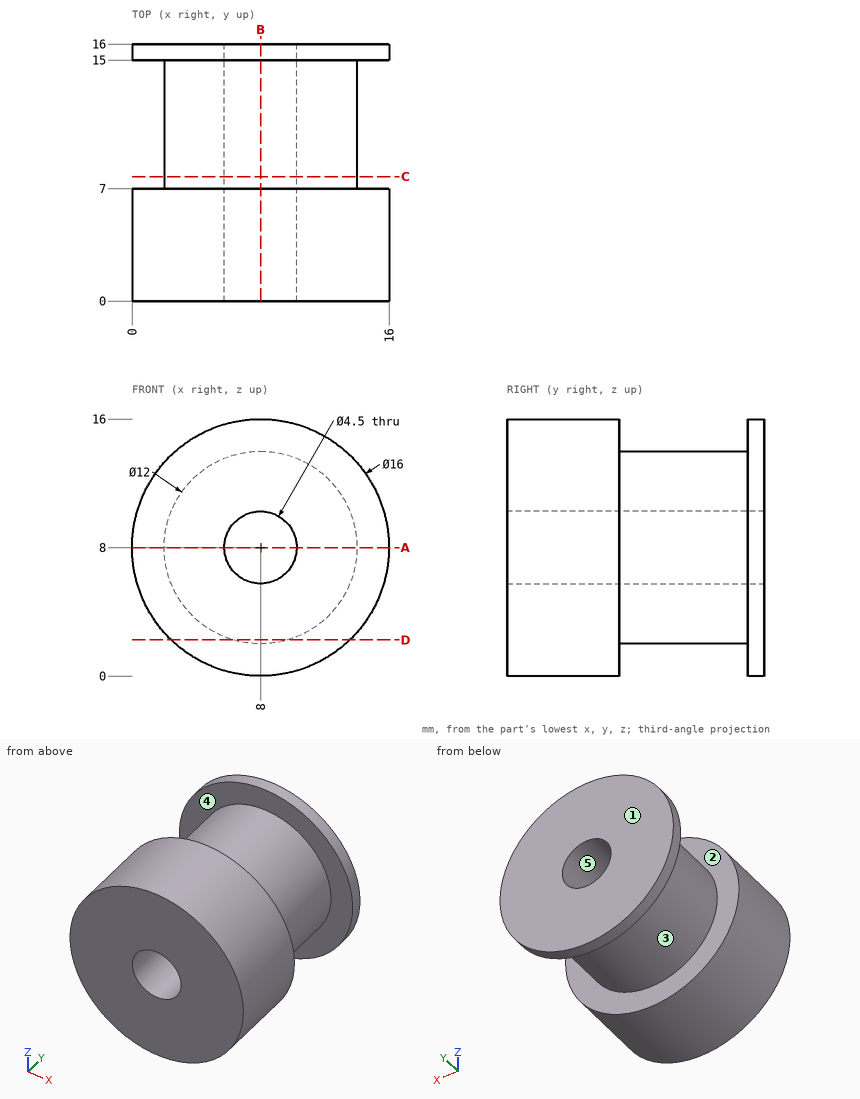
Verification items for this drawing (mm, ordinates from the low corner). A direction names the side the tool comes from. Give positions to 0.01 mm unless a question says otherwise; leave off trailing zeros. Write each loop counter-clockwise with the first axis right and the second up, starting at its lowest first coordinate (ties: lowest second). Pieces come first, ordered by that corner, then holes.
1) Section check C-C, the plane y = 7.75. Record the boundary of the cut face in (x, z).
2) Section check B-B, the plane x = 8. Record the boundary of the cut face in (y, z), and give its area (3 significant figures).
3) Material ranges on L1, parallel to Y at x = 5, z = 14.75; L2, parallel to X at y = 5, z = 8; L3, parallel to X at y = 10.5, z = 8, recorded low to high.
4) Section check D-D, the plane z = 2.25. Record the boundary of the cut face in (x, y).
5) Gauge pin test, flat ends, axial feed: pin 1 (1.5 mm diameter, centred on y = 8, z = 4, fed in from -X); pin 2 (1 mm diameter, centred on y = 9, z = 10, fed in from -X); pin 3 (4 mm diameter, centred on y = 3, z = 2, fed in from +X). Record the tip position at first contact, or that the pin passes through.
6) Access from +Z, -Z, +X, -X, +Y, -Y to the whole of each face (thin tool, end or side, straight path). Record for the marked faces 1 and 2.
7) Release check for a two-part mould opening along X. For the marked faces 3, 4 and 5 record: pulls with the +X half, pulls with the -X half, needs draft (parallel to the pull), parting line crosses it, or undercut.
8) Section check A-A, the plane z = 8. Record the boundary of the cut face in (x, y), and give its area (3 significant figures).
Computed:
1. outline: circle Ø12 at (8, 8); hole circle Ø4.5 at (8, 8)
2. outline: (0, 0) - (7, 0) - (7, 2) - (15, 2) - (15, 0) - (16, 0) - (16, 5.75) - (0, 5.75) - close; (0, 10.25) - (16, 10.25) - (16, 16) - (15, 16) - (15, 14) - (7, 14) - (7, 16) - (0, 16) - close
2. area: 152 mm2
3. L1: y = 0 to 7, 15 to 16
3. L2: x = 0 to 5.75, 10.25 to 16
3. L3: x = 2 to 5.75, 10.25 to 14
4. outline: (2.44, 0) - (13.56, 0) - (13.56, 7) - (9.71, 7) - (9.71, 15) - (13.56, 15) - (13.56, 16) - (2.44, 16) - (2.44, 15) - (6.29, 15) - (6.29, 7) - (2.44, 7) - close
5. pin 1: stops at x = 2.96
5. pin 2: stops at x = 2.19
5. pin 3: stops at x = 14.93
6. face 1: +Z, -Z, +X, -X, +Y
6. face 2: none
7. face 3: parting line crosses it
7. face 4: needs draft
7. face 5: undercut
8. outline: (0, 0) - (5.75, 0) - (5.75, 16) - (0, 16) - (0, 15) - (2, 15) - (2, 7) - (0, 7) - close; (10.25, 0) - (16, 0) - (16, 7) - (14, 7) - (14, 15) - (16, 15) - (16, 16) - (10.25, 16) - close
8. area: 152 mm2
